from build123d import *

# Parameters (mm, degrees)
F1_DEPTH = 609.6
F3_D     = 2.54


with BuildPart() as f1:
    # F0 (on Front) → F1 (new body)
    with BuildSketch(Plane.XZ):
        with BuildLine():
            Line((-6.559787, -4.439499), (-11.639787, -4.439499))
            Line((-11.639787, -4.439499), (-11.639787, -11.043499))
            Line((-11.639787, -11.043499), (-4.019787, -11.043499))
            Line((-4.019787, -11.043499), (-4.019787, -16.123499))
            Line((-4.019787, -16.123499), (-8.575975, -18.370174))
            Line((-8.575975, -18.370174), (-8.575975, -20.656174))
            Line((-8.575975, -20.656174), (-4.765975, -20.656174))
            Line((-4.765975, -20.656174), (-4.155417, -20.148174))
            Line((-4.155417, -20.148174), (2.194583, -20.148174))
            Line((2.194583, -20.148174), (2.854025, -20.59087))
            Line((2.854025, -20.59087), (6.664025, -20.59087))
            Line((6.664025, -20.59087), (6.664025, -18.30487))
            Line((6.664025, -18.30487), (2.076213, -16.123499))
            Line((2.076213, -16.123499), (2.076213, -11.043499))
            Line((2.076213, -11.043499), (9.696213, -11.043499))
            Line((9.696213, -11.043499), (9.696213, -4.439499))
            Line((9.696213, -4.439499), (4.616213, -4.439499))
            Line((4.616213, -4.439499), (3.473213, -5.113759))
            Line((3.473213, -5.113759), (-3.702287, -5.113759))
            ThreePointArc((-3.702287, -5.113759), (-4.146787, -5.558259), (-4.591287, -5.113759))
            Line((-4.591287, -5.113759), (-5.416787, -5.113759))
            Line((-5.416787, -5.113759), (-6.559787, -4.439499))
        make_face()
    extrude(amount=F1_DEPTH)

    # F3 (through all)
    with Locations(Plane.XY.offset(-5.113759)):
        with Locations((0, -33.02), (0, -92.71), (0, -152.4), (0, -212.09), (0, -272.464672), (0, -331.47), (0, -391.16), (0, -450.85), (0, -540.461149)):
            Hole(F3_D / 2)


solid = f1.part
The model under review builds one solid part; all positions refer to its coordinate system, in mm. Round coordinates to 2 decimals unless told otherwise and drop trailing zeros. Loops run counter-clockwise (first coordinate to the right, second up) from the corner with the lowest first, then second, coordinate; pieces in that order, holes last. Notation, with made-up numbers: M -14,37.5 L 27,37.5 A27 ccw 27,69.5 Z; hole C -38.75,23 d2. An arc over 180 degrees is marked long. Answer as CSV lines item,"result". Start each with the question number.
Item 1: Insertion check: P1, Ø2.5, axis at y = -449.5, z = -19, coming from the -X side; P2, Ø8, axis at x = 0, y = -452.5, coming from the -Z side; P3, Ø3, axis at x = 0, y = -212.09, coming from the -Z side. Each pin has a flat end and moves straight along its axis. Give the tip position at first contact, or say it passes through.
Item 2: Consider section A-A (y = -197). Write out the cut boundary in (x, z).
Item 3: Wall thickness on line 1 (X direction, y = -33, z = -15); line 2 (Z direction, x = 6.5, y = -514); line 3 (Z direction, x = 9, y = -331): over which ranges is each line inside the solid? List them lowest first. Write a range as [from, to].
Answer:
1,P1,"stops at x = -8.58"
1,P2,"stops at z = -20.59"
1,P3,"stops at z = -20.15"
2,outline,"M -11.64,-11.04 L -4.02,-11.04 L -4.02,-16.12 L -8.58,-18.37 L -8.58,-20.66 L -4.77,-20.66 L -4.16,-20.15 L 2.19,-20.15 L 2.85,-20.59 L 6.66,-20.59 L 6.66,-18.3 L 2.08,-16.12 L 2.08,-11.04 L 9.7,-11.04 L 9.7,-4.44 L 4.62,-4.44 L 3.47,-5.11 L -3.7,-5.11 A0.44 cw -4.59,-5.11 L -5.42,-5.11 L -6.56,-4.44 L -11.64,-4.44 Z"
3,line 1,"x = [-4.02, -1.27], [1.27, 2.08]"
3,line 2,"z = [-20.59, -18.23], [-11.04, -4.44]"
3,line 3,"z = [-11.04, -4.44]"
